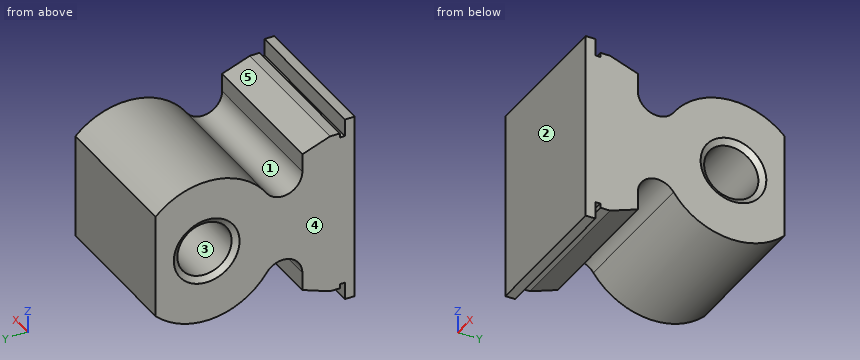
```python
from build123d import *

# Parameters (mm, degrees)
BODYSKE_R    = 1.65
BODY_DEPTH   = 8.9
TOPCUTSKE_W  = 8.89
TOPCUTSKE_H  = 8.89
TOPCUT_DEPTH = 8.9


with BuildPart() as part:
    # BodySke → Body (new body)
    with BuildSketch(Plane(origin=(0, 0, 0), x_dir=(0, 0, -1), z_dir=(1, 0, 0))):
        with BuildLine():
            Line((-5.74, -9), (5.74, -9))
            Line((5.74, -9), (5.74, -8.4))
            Line((5.74, -8.4), (4.686666667, -8.4))
            Line((4.686666667, -8.4), (4.686666667, -8.1))
            Line((4.686666667, -8.1), (4.95, -8.1))
            Line((4.95, -8.1), (4.95, -7.5))
            Line((4.95, -7.5), (4.338530006, -5.82))
            Line((4.338530006, -5.82), (3.223696854, -5.82))
            ThreePointArc((3.223696854, -5.82), (2.08483996, -4.983958225), (2.54124896, -3.646927299))
            ThreePointArc((2.54124896, -3.646927299), (0, 4.445), (-2.54124896, -3.646927299))
            ThreePointArc((-2.54124896, -3.646927299), (-2.08483996, -4.983958225), (-3.223696854, -5.82))
            Line((-3.223696854, -5.82), (-4.338530006, -5.82))
            Line((-4.338530006, -5.82), (-4.95, -7.5))
            Line((-4.95, -7.5), (-4.95, -8.1))
            Line((-4.95, -8.1), (-4.686666667, -8.1))
            Line((-4.686666667, -8.1), (-4.686666667, -8.4))
            Line((-4.686666667, -8.4), (-5.74, -8.4))
            Line((-5.74, -8.4), (-5.74, -9))
        make_face()
        Circle(BODYSKE_R, mode=Mode.SUBTRACT)
    extrude(amount=BODY_DEPTH)

    # EndChamferSke → EndChamfer (revolve, cut)
    with BuildSketch(Plane.XY, mode=Mode.PRIVATE) as endchamfer_sk:
        Polygon((-0.254, 2), (0.00254, 2), (0.247521613, 1.65), (-0.254, 1.65), align=None)
        Polygon((9.154, 2), (8.89746, 2), (8.652478387, 1.65), (9.154, 1.65), align=None)
    revolve(endchamfer_sk.sketch.rotate(Axis((-5.105879624, 0, 0), (1, 0, 0)), 90), axis=Axis((-5.105879624, 0, 0), (1, 0, 0)), mode=Mode.SUBTRACT)

    # TopCutSke → TopCut (cut)
    with BuildSketch(Plane.ZY):
        with Locations((0, 7.5565)):
            Rectangle(TOPCUTSKE_W, TOPCUTSKE_H)
    extrude(amount=-TOPCUT_DEPTH, mode=Mode.SUBTRACT)


solid = part.part
```
Build history of the part. All positions in model axes, mm. Face numbers are marked on the shaded views. A direction names the side the tool comes from. Give positions to 0.01 mm unless a question says otherwise; leave off trailing zeros. Loops run counter-clockwise (first coordinate to the right, second up) from the corner with the lowest first, then second, coordinate; pieces in that order, holes last.
Item 1: Drill centre lines: line 1 (Y direction, x = 2, z = 0); line 2 (Z direction, x = 8, y = -8); line 3 (Y direction, x = 3.5, z = -4). Where is each one in solid material? Low to high.
Answers follow:
line 1: y = -9 to -1.65, 1.65 to 3.11
line 2: z = -4.95 to 4.95
line 3: y = -9 to -5.82, -1.94 to 1.94
Item 2: Pull direction Z, two halves, no side cores. Call the marked faces 1, 2 and 3: released by +Z, released by -Z, zero draft, split by the parting line, or undercut.
Answers follow:
face 1: released by +Z
face 2: zero draft
face 3: undercut
Item 3: Flat gauge pins, fed straight in: pin 1 (0.7 mm diameter, centred on x = 4.5, y = -7.5, fed in from +Z); pin 2 (4 mm diameter, centred on x = 4.5, y = -4.5, fed in from +Z). Where does each tip first touch, or does it go through?
Answers follow:
pin 1: stops at z = 4.95
pin 2: stops at z = 4.59
Item 4: Slice it at D-D, the plane z = 3. List the corners of the cut face in (x, y).
Answers follow:
outline: (0, -9) - (8.9, -9) - (8.9, -5.8) - (0, -5.8) - close; (0, -3.28) - (8.9, -3.28) - (8.9, 3.11) - (0, 3.11) - close
Item 5: Which spindle directions (+Z, -Z, +X, -X, +Y, -Y) get a long thin tool onto all of the face, cutting with end or side? Do the marked faces 4 and 5. Say none if no direction does.
Answers follow:
face 4: +Z, -Z, -X, +Y, -Y
face 5: +Z, +X, -X
